Design review of the part built by this model. Coordinates are the model's own, in mm. Give positions to 0.01 mm unless a question says otherwise; leave off trailing zeros. Order: outer loops, then holes, each group sorted by start corner. A loop starts at its lowest first (then second) coordinate and runs counter-clockwise, first axis right, second up. Notation, with made-up numbers: M 24,-19 L 39,-19 A11 ccw 39,0 Z; hole C 55.25,-13.5 d7. An arc over 180 degrees is marked long. Answer as a JSON object with one key per item and string values.
from build123d import *

# Parameters (mm, degrees)
SKETCH2_R           = 2.48
BOSS_EXTRUDE1_DEPTH = 10
BOSS_EXTRUDE1_TAPER = 2


with BuildPart() as part:
    # Sketch1 → Revolve1 (revolve)
    with BuildSketch(Plane(origin=(0, 0, 0), x_dir=(1, 0, 0), z_dir=(0, 1, 0))):
        with BuildLine():
            Line((0, 2.48), (0, -2.48))
            ThreePointArc((0, -2.48), (2.48, 0), (0, 2.48))
        make_face()
    revolve(axis=Axis((0, 0, -2.48), (0, 0, 1)))

    # Sketch2 → Boss-Extrude1 (add)
    with BuildSketch(Plane(origin=(0, 0, 0), x_dir=(1, 0, 0), z_dir=(0, 1, 0))):
        Circle(SKETCH2_R)
    extrude(amount=BOSS_EXTRUDE1_DEPTH, taper=BOSS_EXTRUDE1_TAPER)

    # Sketch3 → Revolve2 (revolve)
    with BuildSketch(Plane(origin=(0, 10, 0), x_dir=(1, 0, 0), z_dir=(0, 1, 0))):
        with BuildLine():
            Line((0, 2.130792305), (0, -2.130792305))
            ThreePointArc((0, -2.130792305), (2.130792305, 0), (0, 2.130792305))
        make_face()
    revolve(axis=Axis((0, 10, -2.130792305), (0, 0, 1)))


solid = part.part
(1) We need section A-A (x = 0). Write out the cut boundary in (y, z), plus the area to 3 significant figures.
Checked values:
{"outline": "M 0.17,-2.47 L 10,-2.13 A2.13 ccw 10,2.13 L 0.17,2.47 A2.48 ccw long Z", "area": "62.9 mm^2"}
(2) Insertion check: pin 1 (1 mm diameter, centred on x = -0.5, z = 1, fed in from +Y); pin 2 (2 mm diameter, centred on x = 1.5, z = -1.5, fed in from -Y); pin 3 (2 mm diameter, centred on y = 2, z = 1.5, fed in from +X). Each pin has a flat end and moves straight along its axis. Give the tip position at first contact, or say it passes through.
Checked values:
{"pin 1": "stops at y = 12.04", "pin 2": "stops at y = -2.21", "pin 3": "stops at x = 2.36"}
(3) We need section B-B (y = -1). Write out the cut boundary in (x, z), plus the area to 3 significant figures.
Checked values:
{"outline": "C 0,0 d4.54", "area": "16.2 mm^2"}
(4) We need section C-C (y = 3). Write out the cut boundary in (x, z), plus the area to 3 significant figures.
Checked values:
{"outline": "C 0,0 d4.75", "area": "17.7 mm^2"}
(5) To check wall thickness, follow L1, parallel to Y at x = 1.8, z = 0.8; L2, parallel to Z at x = -1.5, y = -0.25; L3, parallel to Z at x = 1.75, y = 8.5. State the ranges of each line that lie inside material, in increasing order. Write a range as from..to.
Checked values:
{"L1": "y = -1.51..10.81", "L2": "z = -1.96..1.96", "L3": "z = -1.31..1.31"}
